from build123d import *

# Parameters (mm, degrees)
SKETCH1_R           = 11
BOSS_EXTRUDE1_DEPTH = 1.375


with BuildPart() as part:
    # Sketch1 → Boss-Extrude1 (new, symmetric)
    with BuildSketch(Plane(origin=(0, 0, 0), x_dir=(1, 0, 0), z_dir=(0, 1, 0))):
        with Locations(Location((0, 0, 0), (0, 0, 270))):
            Circle(SKETCH1_R)
        with BuildLine():
            Line((-5, 3.31662479), (-5, -3.31662479))
            ThreePointArc((-5, -3.31662479), (0, -6), (5, -3.31662479))
            Line((5, -3.31662479), (5, 3.31662479))
            ThreePointArc((5, 3.31662479), (0, 6), (-5, 3.31662479))
        make_face(mode=Mode.SUBTRACT)
    extrude(amount=BOSS_EXTRUDE1_DEPTH, both=True)


solid = part.part
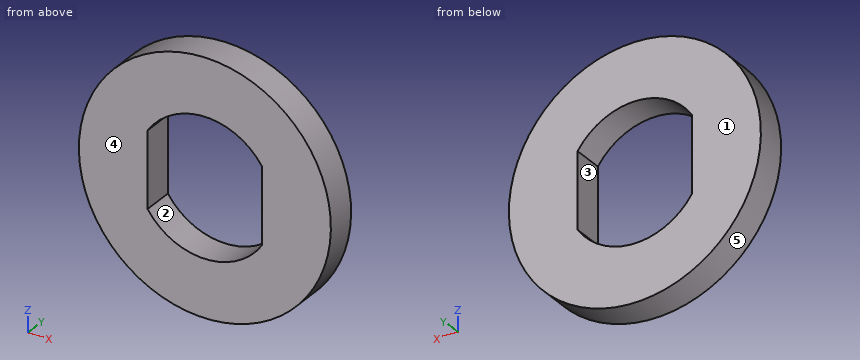
Could you check a few things on this model? Use its own coordinates, in mm. Face numbers are marked on the shaded views. A direction names the side the tool comes from. Give positions to 0.01 mm unless a question says otherwise; leave off trailing zeros. Loops run counter-clockwise (first coordinate to the right, second up) from the corner with the lowest first, then second, coordinate; pieces in that order, holes last. Notation, with made-up numbers: (-35, -5.75) -> (8, -5.75) arc R29 ccw to (8, 28.25) -> close; hole circle Ø1 at (43, 32). An arc over 180 degrees is marked (long way). Answer as CSV lines item,"result". Start each with the question number.
(1) If we section it at B-B on x = 0: Write out the boundary of the cut face in (y, z) (3 decimals).
(2) If we section it at A-A on z = 0: Write out the boundary of the cut face in (x, y) (3 decimals), then the cut area to 3 significant figures.
(3) If we section it at D-D on z = -7.25: Write out the boundary of the cut face in (x, y) (3 decimals).
(4) I'm going to push flat-ended pins straight in: pin 1 Ø1.4 at (y, z) = (0.5, -1) entering from -X; pin 2 Ø1.5 at (y, z) = (-1, -7.5) entering from +X; pin 3 Ø1 at (x, y) = (7, -1) entering from -Z. Where does each tip first touch, or does it pass through?
(5) If we section it at C-C on y = 0.95: Write out the boundary of the cut face in (x, z).
(6) I need wall thicknesses on probe 1 along Z at (x, y) = (-4.75, 0.4); probe 2 along X at (y, z) = (-0.35, 4.5); probe 3 along Z at (x, y) = (3.25, 0.5). Which ranges of each line are inside material? Lowest first, please.
(7) Which directions (+Z, -Z, +X, -X, +Y, -Y) give clear straight access to the entire face, cutting with the end or side of a thin tool? Please do the marked faces 1 and 2.
(8) We'd pull the mould along Z, two halves only. Please class the marked faces 3, 4 and 5: released by +Z, released by -Z, zero draft, split by the parting line, or undercut.
Computed:
1,outline,"(-1.375, -11) -> (1.375, -11) -> (1.375, -6) -> (-1.375, -6) -> close; (-1.375, 6) -> (1.375, 6) -> (1.375, 11) -> (-1.375, 11) -> close"
2,outline,"(-11, -1.375) -> (-5, -1.375) -> (-5, 1.375) -> (-11, 1.375) -> close; (5, -1.375) -> (11, -1.375) -> (11, 1.375) -> (5, 1.375) -> close"
2,area,"33.0 mm2"
3,outline,"(-8.273, -1.375) -> (8.273, -1.375) -> (8.273, 1.375) -> (-8.273, 1.375) -> close"
4,pin 1,"stops at x = -11"
4,pin 2,"stops at x = 8.69"
4,pin 3,"stops at z = -8.87"
5,outline,"circle Ø22 at (0, 0); hole (-5, -3.32) arc R6 ccw to (5, -3.32) -> (5, 3.32) arc R6 ccw to (-5, 3.32) -> close"
6,probe 1,"z = -9.92 to -3.67, 3.67 to 9.92"
6,probe 2,"x = -10.04 to -3.97, 3.97 to 10.04"
6,probe 3,"z = -10.51 to -5.04, 5.04 to 10.51"
7,face 1,"+Z, -Z, +X, -X, +Y"
7,face 2,"+Y, -Y"
8,face 3,"undercut"
8,face 4,"zero draft"
8,face 5,"split by the parting line"
